CAD build for the part. Positions are in the model's coordinates, mm. A direction names the side the tool comes from. Coordinates: 2 decimals unless noted, no trailing zeros. Write each loop counter-clockwise with the first axis right and the second up, starting at its lowest first coordinate (ties: lowest second). Pieces come first, ordered by that corner, then holes.
```python
from build123d import *

# Parameters (mm, degrees)
SKETCH_R           = 30
PAD_DEPTH          = 35
SKETCH001_R        = 9.75
POCKET_DEPTH       = 5.5
POCKET001_DEPTH    = 3.5
SKETCH003_R        = 1.75
POCKET002_DEPTH    = 26.001
PAD001_DEPTH       = 9
SKETCH006_R        = 36.546669
SKETCH006_R_2      = 16.734949
POCKET003_DEPTH    = 15
SKETCH008_R        = 11.576804
POCKET004_DEPTH    = 218.576598
POLARPATTERN_COUNT = 6
CHAMFER_SIZE       = 4
CHAMFER001_SIZE    = 2
SKETCH009_R        = 3
POCKET005_DEPTH    = 23
CHAMFER002_SIZE    = 2
CHAMFER003_SIZE    = 8


with BuildPart() as part:
    # Sketch → Pad (new body)
    with BuildSketch(Plane.XY):
        Circle(SKETCH_R)
    extrude(amount=PAD_DEPTH)

    # Sketch001 (on Face3 of Pad) → Pocket (cut)
    with BuildSketch(Plane.XY.offset(35)):
        Circle(SKETCH001_R)
    extrude(amount=-POCKET_DEPTH, mode=Mode.SUBTRACT)

    # Sketch002 (on Face5 of Pocket) → Pocket001 (cut)
    with BuildSketch(Plane.XY.offset(29.5)):
        with BuildLine():
            Line((2.45, -2.839014), (2.45, 2.839014))
            ThreePointArc((2.45, 2.839014), (0, 3.75), (-2.45, 2.839014))
            Line((-2.45, -2.839014), (-2.45, 2.839014))
            ThreePointArc((-2.45, -2.839014), (0, -3.75), (2.45, -2.839014))
        make_face()
    extrude(amount=-POCKET001_DEPTH, mode=Mode.SUBTRACT)

    # Sketch003 (on Face10 of Pocket001) → Pocket002 (cut, through all)
    with BuildSketch(Plane.XY.offset(26)):
        Circle(SKETCH003_R)
    extrude(amount=-POCKET002_DEPTH, mode=Mode.SUBTRACT)

    # Sketch004 (on Face3 of Pocket002) → Pad001 (join)
    with BuildSketch(Plane.XY.offset(35)):
        Polygon((-6.5, 10.255921), (-6.5, 0.5), (-12.416934, 0.5), align=None)
        Polygon((0.5, -6.5), (0.5, -15.116689), (10.696822, -6.5), align=None)
    extrude(amount=-PAD001_DEPTH)

    # Sketch006 (on Face3 of Pad001) → Pocket003 (cut)
    with BuildSketch(Plane.XY.offset(35)):
        Circle(SKETCH006_R)
        Circle(SKETCH006_R_2, mode=Mode.SUBTRACT)
    extrude(amount=-POCKET003_DEPTH, mode=Mode.SUBTRACT)

    # Sketch008 (on Face2 of Pocket003) → Pocket004 (cut, through all)
    with BuildSketch(Plane(origin=(0, 0, 0), x_dir=(1, 0, 0), z_dir=(0, 0, -1))):
        with Locations((0, 36.523853)):
            Circle(SKETCH008_R)
    pocket004 = extrude(amount=-POCKET004_DEPTH, mode=Mode.SUBTRACT)

    # PolarPattern: Pocket004 ×6 about axis
    polarpattern_axis = Axis((0, 0, 0), (0, 0, -1))
    for i in range(1, POLARPATTERN_COUNT):
        add(pocket004.rotate(polarpattern_axis, i * 360 / POLARPATTERN_COUNT), mode=Mode.SUBTRACT)

    # Chamfer
    chamfer_edges = [part.edges().sort_by_distance(p)[0] for p in [
        (15, -25.980762, 0),
        (-15, -25.980762, 0),
        (-30, 0, 0),
        (-15, 25.980762, 0),
        (15, 25.980762, 0),
        (29.795478, 3.497065, 0),
    ]]
    chamfer(chamfer_edges, length=CHAMFER_SIZE)

    # Chamfer001
    chamfer001_edges = [part.edges().sort_by_distance(p)[0] for p in [
        (29.795478, -3.497065, 20),
        (15, -25.980762, 20),
        (15, 25.980762, 20),
        (-15, 25.980762, 20),
        (-15, -25.980762, 20),
        (-30, 0, 20),
    ]]
    chamfer(chamfer001_edges, length=CHAMFER001_SIZE)

    # Sketch009 (on Face10 of Chamfer001) → Pocket005 (cut)
    with BuildSketch(Plane(origin=(0, 0, 0), x_dir=(1, 0, 0), z_dir=(0, 0, -1))):
        Circle(SKETCH009_R)
    extrude(amount=-POCKET005_DEPTH, mode=Mode.SUBTRACT)

    # Chamfer002
    chamfer002_edges = [part.edges().sort_by_distance(p)[0] for p in [
        (-3, 0, 0),
    ]]
    chamfer(chamfer002_edges, length=CHAMFER002_SIZE)

    # Chamfer003
    chamfer003_edges = [part.edges().sort_by_distance(p)[0] for p in [
        (-16.734949, 0, 20),
    ]]
    chamfer(chamfer003_edges, length=CHAMFER003_SIZE)


solid = part.part
```
Item 1: Flat gauge pins, fed straight in: pin 1 Ø1.8 at (x, y) = (0, 1.5) entering from -Z; pin 2 Ø1.5 at (y, z) = (-1, 14.5) entering from -X; pin 3 Ø3 at (x, z) = (-11.5, 13.5) entering from -Y; pin 4 Ø6 at (x, y) = (8.5, 14) entering from -Z. Where does each tip first touch, or does it go through?
Item 2: Which spindle directions (+Z, -Z, +X, -X, +Y, -Y) get a long thin tool onto all of the face, cutting with end or side? Do faces 5 (the flat face through (-15, -20, 20)), 6 (the cylindrical face through (-3, 0, 12)), 7 (the cylindrical face through (14.915, -26.03, 10.902)). Say none if no direction does.
Item 3: Saw through at B-B, the plane z = 10.5. Write the cut outline in (x, y).
Item 4: Saw through at A-A, the plane z = 31.5. Write the cut outline in (x, y), and give its area (3 significant figures).
Item 5: Saw through at C-C, the plane z = 27. Write the cut outline in (x, y).
Item 6: Two-plate mould, pull along X, no slides. Class faces 1 (the flat face through (4, -6.5, 32)), 2 (the conical face through (13.89, 23.77, 1.53)), 3 (the flat face through (0, 2, 23)), 4 (the conical face through (-29, 0, 19)): +X half, -X half, draft (parallel to the pull), parting line (faces both ways), or undercut.
Item 7: Wall check: line 1 along Y through (x, z) = (0, 14.75); line 2 along Z through (x, y) = (-1.5, -5.5); line 3 along Y through (x, z) = (0.5, 9.5). Give the ranges that are in metal, low to high.
Working result:
1. pin 1: stops at z = 23
1. pin 2: stops at x = -30
1. pin 3: stops at y = -28.28
1. pin 4: stops at z = 0
2. face 5: +Z
2. face 6: -Z
2. face 7: +Z, -Z, +X, -Y
3. outline: (-29.18, -6.95) arc R11.58 cw to (-20.61, -21.8) arc R30 ccw to (-8.58, -28.75) arc R11.58 cw to (8.58, -28.75) arc R30 ccw to (20.61, -21.8) arc R11.58 cw to (29.18, -6.95) arc R30 ccw to (29.18, 6.95) arc R11.58 cw to (20.61, 21.8) arc R30 ccw to (8.58, 28.75) arc R11.58 cw to (-8.58, 28.75) arc R30 ccw to (-20.61, 21.8) arc R11.58 cw to (-29.18, 6.95) arc R30 ccw to start; hole circle Ø6 at (0, 0)
4. outline: circle Ø33.47 at (0, 0); hole (-9.74, 0.5) arc R9.75 ccw to (0.5, -9.74) - (0.5, -6.5) - (7.27, -6.5) arc R9.75 ccw to (-6.5, 7.27) - (-6.5, 0.5) - close
4. area: 611 mm2
5. outline: circle Ø35.47 at (0, 0); hole (-2.45, -2.84) arc R3.75 ccw to (2.45, -2.84) - (2.45, 2.84) arc R3.75 ccw to (-2.45, 2.84) - close
6. face 1: undercut
6. face 2: +X half
6. face 3: undercut
6. face 4: -X half
7. line 1: y = -24.95 to -3, 3 to 24.95
7. line 2: z = 0 to 29.5
7. line 3: y = -24.96 to -2.96, 2.96 to 24.96
